Autodesk Inventor part; units mm, degrees
ref_plane "YZ Plane" through (0, 0, 0) normal (1, 0, 0) x (0, 1, 0)
ref_plane "XZ Plane" through (0, 0, 0) normal (0, 1, 0) x (-1, 0, 0)
ref_plane "XY Plane" through (0, 0, 0) normal (0, 0, 1) x (1, 0, 0)
sketch "Esquisse1" plane through (0, 0, 0) normal (0, 1, 0) x (-1, 0, 0)
  line L0 (6.5, 15) -> (-6.5, 15)
  line L1 (-6.5, 15) -> (-6.5, -15)
  line L2 (-6.5, -15) -> (6.5, -15)
  line L3 (6.5, -15) -> (6.5, 15)
  line L4 (4, 15) -> (-4, 15)
  line L5 (-4, 15) -> (-4, 22.5)
  line L6 (-4, 22.5) -> (4, 22.5)
  line L7 (4, 22.5) -> (4, 15)
  line L8 (4, -15) -> (-4, -15)
  line L9 (-4, -15) -> (-4, -22.5)
  line L10 (-4, -22.5) -> (4, -22.5)
  line L11 (4, -22.5) -> (4, -15)
  line L12 (-6.5, -5) -> (-12, -5)
  line L13 (-12, -5) -> (-12, 5)
  line L14 (-12, 5) -> (-6.5, 5)
  line L15 (-6.5, 5) -> (-6.5, -5)
  point P0 (0, 0)
  dimension "d0" = 30
  dimension "d1" = 15
  dimension "d2" = 13
  dimension "d3" = 6.5
  dimension "d4" = 45
  dimension "d5" = 22.5
  dimension "d6" = 8
  dimension "d7" = 4
  dimension "d8" = 5.5
  dimension "d9" = 10
  dimension "d10" = 5
extrude "Extrusion1" add sketch "Esquisse1" along normal blind 1
sketch "Esquisse2" plane through (0, 1, 0) normal (0, 1, 0) x (1, 0, 0)
  line L0 (-6.5, -15) -> (6.5, -15)
  line L1 (6.5, -15) -> (6.5, 15)
  line L2 (6.5, 15) -> (-6.5, 15)
  line L3 (-6.5, 15) -> (-6.5, -15)
  point P0 (0, 0)
extrude "Extrusion2" add sketch "Esquisse2" along normal blind 12
sketch "Esquisse3" plane through (0, 0, 0) normal (0, -1, 0) x (1, 0, 0)
  line L0 (-4, 22.5) -> (4, 22.5) construction
  line L1 (4, 22.5) -> (4, 15) construction
  line L2 (4, 15) -> (-4, 15) construction
  line L3 (-4, 15) -> (-4, 22.5) construction
  line L4 (-4, -15) -> (4, -15) construction
  line L5 (4, -15) -> (4, -22.5) construction
  line L6 (4, -22.5) -> (-4, -22.5) construction
  line L7 (-4, -22.5) -> (-4, -15) construction
  line L8 (-4, 15) -> (4, 22.5) construction
  line L9 (4, 15) -> (-4, 22.5) construction
  line L10 (-4, -22.5) -> (4, -15) construction
  line L11 (-4, -15) -> (4, -22.5) construction
  circle A0 centre (0, -18.75) radius 1.5
  circle A1 centre (0, 18.75) radius 1.5
  point P0 (0, 0)
  dimension "d15" = 3
  dimension "d16" = 3
extrude "Extrusion3" cut sketch "Esquisse3" against normal through all
equation "\"d16\" = d15"
properties part number "gp2"
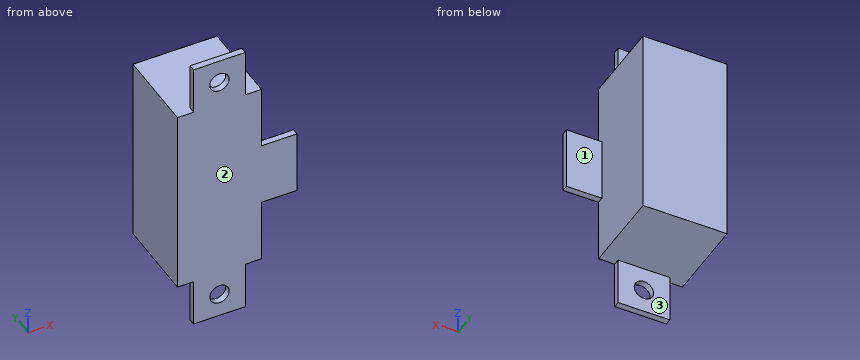
The listing builds one solid part. Answer for the finished solid, in the listing's coordinates (mm). Face numbers are marked on the shaded views. A direction names the side the tool comes from. Round coordinates to 2 decimals unless told otherwise and drop trailing zeros. Order: outer loops, then holes, each group sorted by start corner. A loop starts at its lowest first (then second) coordinate and runs counter-clockwise, first axis right, second up. Notation, with made-up numbers: M 34,73.25 L 77,73.25 A6 cw 77,78.25 Z; hole C -4,22 d3. An arc over 180 degrees is marked long. Answer in a Markdown table with one row per item. Add a question column.
1) The part is cut by section D-D on y = 7.5. Determine the outline of the cut face in (x, z), plus the area to 3 significant figures.
2) Consider line 1 along Z through (x, y) = (0, 0.5); line 2 along Z through (x, y) = (-2, 12.5); line 3 along X through (y, z) = (10.5, 3.5). Determine where each line is inside the solid, lowest interval first. Write a range as from..to.
3) Which of the six approach directions +Z, -Z, +X, -X, +Y, -Y give full straight-line access (tool end or side, diameter ignored) to the marked faces 1, 2 and 3?
4) The part is cut by section C-C on z = -4. Determine the outline of the cut face in (x, y), plus the area to 4 significant figures.
5) Flat-ended cylindrical pins translate along their axes: pin 1 Ø3 at (y, z) = (3, 10) entering from +X; pin 2 Ø3 at (x, y) = (-2, 7.5) entering from -Z; pin 3 Ø5 at (x, y) = (2.5, 9) entering from +Z. Find the tip coordinate at first contact, or state that the pin passes through.
6) The part is cut by section A-A on z = -18.75. Determine the outline of the cut face in (x, y), plus the area to 3 significant figures.
7) The part is cut by section B-B on x = 0. Determine the outline of the cut face in (y, z), plus the area to 3 significant figures.
Findings below:
| question | item | result |
|---|---|---|
| 1 | outline | M -6.5,-15 L 6.5,-15 L 6.5,15 L -6.5,15 Z |
| 1 | area | 390 mm² |
| 2 | line 1 | z = -22.5..-20.25, -17.25..17.25, 20.25..22.5 |
| 2 | line 2 | z = -15..15 |
| 2 | line 3 | x = -6.5..6.5 |
| 3 | face 1 | +Z, -Z, +X, +Y |
| 3 | face 2 | +Z, -Z, +X, -X, -Y |
| 3 | face 3 | -Z, +X, -X, +Y |
| 4 | outline | M -6.5,0 L 12,0 L 12,1 L 6.5,1 L 6.5,13 L -6.5,13 Z |
| 4 | area | 174.5 mm² |
| 5 | pin 1 | stops at x = 6.5 |
| 5 | pin 2 | stops at z = -15 |
| 5 | pin 3 | stops at z = 15 |
| 6 | outline | M -4,0 L -1.5,0 L -1.5,1 L -4,1 Z; M 1.5,0 L 4,0 L 4,1 L 1.5,1 Z |
| 6 | area | 5.00 mm² |
| 7 | outline | M 0,-22.5 L 1,-22.5 L 1,-20.25 L 0,-20.25 Z; M 0,-17.25 L 1,-17.25 L 1,-15 L 13,-15 L 13,15 L 1,15 L 1,17.25 L 0,17.25 Z; M 0,20.25 L 1,20.25 L 1,22.5 L 0,22.5 Z |
| 7 | area | 399 mm² |
